Geometry: final body of the model. Coordinates: model frame, mm. Face numbers are marked on the shaded views. Round coordinates to 2 decimals unless told otherwise and drop trailing zeros. Order: outer loops, then holes, each group sorted by start corner. A loop starts at its lowest first (then second) coordinate and runs counter-clockwise, first axis right, second up. Notation, with made-up numbers: (2.5, 46.25) - (39.5, 46.25) arc R22 cw to (39.5, 52.25) - close; hole circle Ø6 at (9.5, 10.25). An arc over 180 degrees is marked (long way). Put each result on its own line as item: value. Start each with the question number.
(1) Section A-A (y = 1.1). Output: boundary loops of the cut face in (x, z) (3 decimals).
(2) Section B-B (x = -18). Output: boundary loops of the cut face in (y, z) (3 decimals).
(3) Section C-C (z = -6.25). Output: boundary loops of the cut face in (x, y) (3 decimals), and give its area (3 significant figures).
(4) Material intervals for L1, parallel to Z at x = -10, y = 0.5 (3 decimals); L2, parallel to Z at x = -16.25, y = 0.95 (3 decimals); L3, parallel to X at y = 1.65, z = -6.5, sorted ascending. Write a range as [from, to].
(5) Pin query (flat end, axial travel): P1, Ø1, axis at x = -9, y = 0.5, coming from the -Z side (3 decimals). Return the tip coordinate at first contact, or that it passes through.
(6) Pull-direction query (Z, two-part tool) for the marked faces 1, 2, 3 and 4; classes: released by +Z, released by -Z, zero draft, split by the parting line, or undercut.
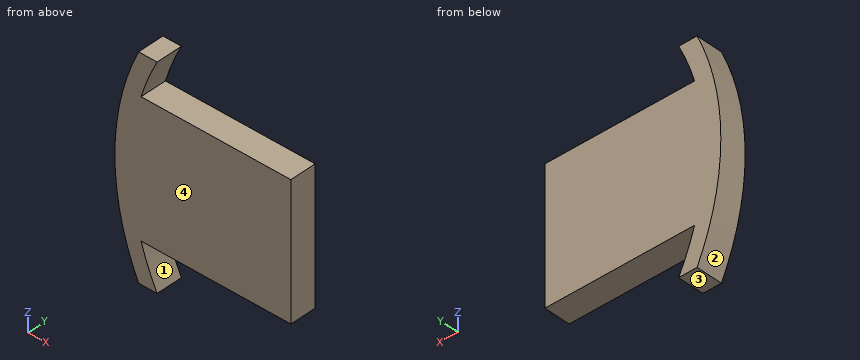
from build123d import *

# Parameters (mm, degrees)
BOSS_EXTRUDE2_DEPTH = 1.975


with BuildPart() as part:
    # Sketch1 → Boss-Extrude2 (new body)
    with BuildSketch(Plane(origin=(0, 0, 0), x_dir=(1, 0, 0), z_dir=(0, 1, 0))):
        with BuildLine():
            ThreePointArc((-16.969439443, 7.975), (-18.75, 0), (-16.969439443, -7.975))
            Line((-16.969439443, -7.975), (-15.582823878, -7.975))
            ThreePointArc((-15.582823878, -7.975), (-16.252359809, -6.502755234), (-16.783158225, -4.975))
            Line((-16.783158225, -4.975), (-5.555, -4.975))
            Line((-5.555, -4.975), (-5.555, 4.975))
            Line((-5.555, 4.975), (-16.783158225, 4.975))
            ThreePointArc((-16.783158225, 4.975), (-16.252359809, 6.502755234), (-15.582823878, 7.975))
            Line((-15.582823878, 7.975), (-16.969439443, 7.975))
        make_face()
    extrude(amount=BOSS_EXTRUDE2_DEPTH)


solid = part.part
Checks:
1. outline: (-16.969, -7.975) - (-15.583, -7.975) arc R17.505 cw to (-16.783, -4.975) - (-5.555, -4.975) - (-5.555, 4.975) - (-16.783, 4.975) arc R17.505 cw to (-15.583, 7.975) - (-16.969, 7.975) arc R18.75 ccw to start
2. outline: (0, -5.25) - (1.975, -5.25) - (1.975, 5.25) - (0, 5.25) - close
3. outline: (-17.678, 0) - (-16.351, 0) - (-16.351, 1.975) - (-17.678, 1.975) - close
3. area: 2.62 mm²
4. L1: z = [-4.975, 4.975]
4. L2: z = [-7.975, -6.509], [-4.975, 4.975], [6.509, 7.975]
4. L3: x = [-17.59, -16.25]
5. P1: stops at z = -4.975
6. face 1: undercut
6. face 2: split by the parting line
6. face 3: released by -Z
6. face 4: zero draft
